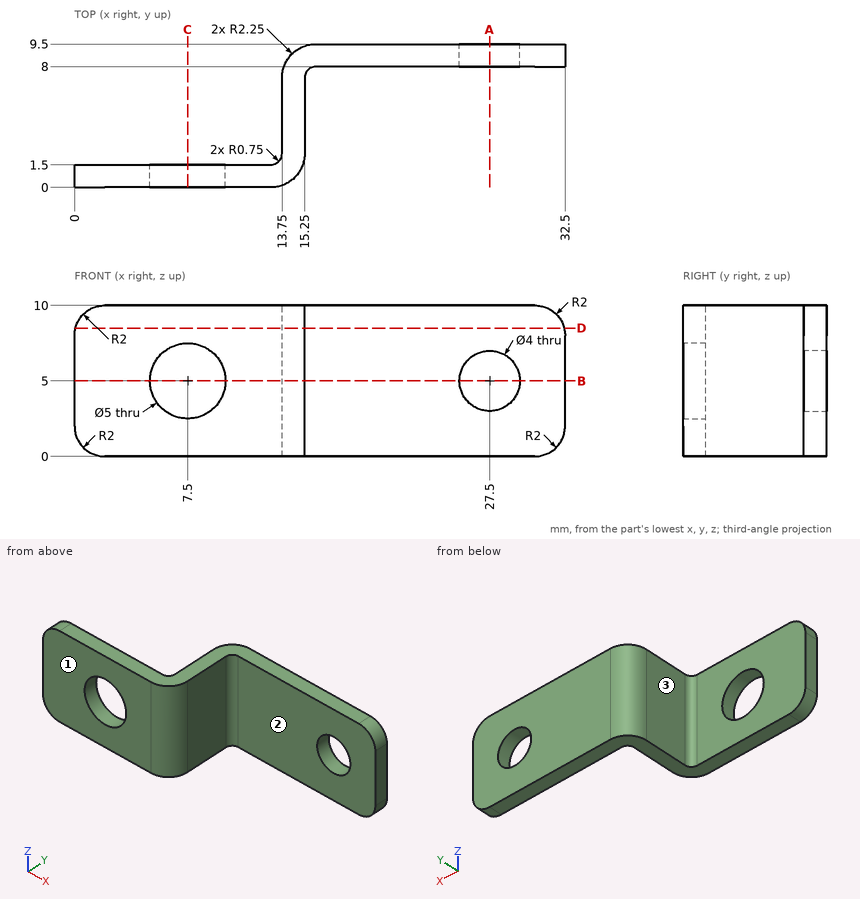
Drawing for the job (mm, zero at the part's lowest x, y, z). A direction names the side the tool comes from. Round coordinates to 2 decimals unless told otherwise and drop trailing zeros. Write each loop counter-clockwise with the first axis right and the second up, starting at its lowest first coordinate (ties: lowest second). Pieces come first, ordered by that corner, then holes. Notation, with made-up numbers: (58, 62.5) - (85, 62.5) arc R30 ccw to (85, 98.5) - close; hole circle Ø11 at (25.25, -21). An arc over 180 degrees is marked (long way). Write item = value, one per line. Start each with the question number.
Q1. Which spindle directions (+Z, -Z, +X, -X, +Y, -Y) get a long thin tool onto all of the face, cutting with end or side? Do the marked faces 1, 2 and 3. Say none if no direction does.
Q2. Drop flat-ended pins along their axis: pin 1 (4.5 mm diameter, centred on x = 27.5, z = 5, fed in from -Y); pin 2 (1.5 mm diameter, centred on y = 3, z = 3, fed in from -X); pin 3 (5 mm diameter, centred on x = 6.5, z = 6.5, fed in from +Y). Give the stop position or say it passes through.
Q3. Band-saw the part on B-B (z = 5). Give the cut face in (x, y), then the cut area to 3 significant figures.
Q4. Band-saw the part on D-D (z = 8.5). Give the cut face in (x, y).
Q5. Band-saw the part on C-C (x = 7.5). Give the cut face in (y, z).
Q6. Probe L1, parallel to X at y = 5.25, z = 4; L2, parallel to Y at x = 27, z = 3; L3, parallel to Y at x = 8.5, z = 9. List the from-to ranges inside material, lowest first. Write a range as from..to.
Q7. Band-saw the part on A-A (x = 27.5). Give the cut face in (y, z).
Answers below:
q1.face_1 = +Z, -Z, +X, -X, -Y
q1.face_2 = +Z, -Z, +X, -Y
q1.face_3 = +Z, -Z, -X, +Y
q2.pin_1 = 8
q2.pin_2 = 13.75
q2.pin_3 = 1.5
q3.outline = (0, 0) - (5, 0) - (5, 1.5) - (0, 1.5) - close; (10, 0) - (13, 0) arc R2.25 ccw to (15.25, 2.25) - (15.25, 7.25) arc R0.75 cw to (16, 8) - (25.5, 8) - (25.5, 9.5) - (16, 9.5) arc R2.25 ccw to (13.75, 7.25) - (13.75, 2.25) arc R0.75 cw to (13, 1.5) - (10, 1.5) - close; (29.5, 8) - (32.5, 8) - (32.5, 9.5) - (29.5, 9.5) - close
q3.area = 45.3 mm2
q4.outline = (0.06, 0) - (13, 0) arc R2.25 ccw to (15.25, 2.25) - (15.25, 7.25) arc R0.75 cw to (16, 8) - (32.44, 8) - (32.44, 9.5) - (16, 9.5) arc R2.25 ccw to (13.75, 7.25) - (13.75, 2.25) arc R0.75 cw to (13, 1.5) - (0.06, 1.5) - close
q5.outline = (0, 0) - (1.5, 0) - (1.5, 2.5) - (0, 2.5) - close; (0, 7.5) - (1.5, 7.5) - (1.5, 10) - (0, 10) - close
q6.L1 = 13.75..15.25
q6.L2 = 8..9.5
q6.L3 = 0..1.5
q7.outline = (8, 0) - (9.5, 0) - (9.5, 3) - (8, 3) - close; (8, 7) - (9.5, 7) - (9.5, 10) - (8, 10) - close
